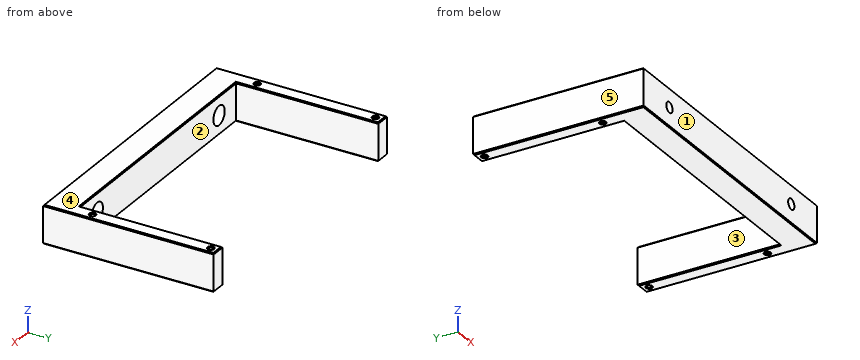
```python
from build123d import *

# Parameters (mm, degrees)
BOSS_EXTRUDE1_DEPTH            = 20
M3X0_5_TAPPED_HOLE1_D          = 2.5
CHAMFER1_SIZE                  = 0.5
CBORE_FOR_M5_SHCS1_D           = 5.5
CBORE_FOR_M5_SHCS1_CBORE_D     = 10
CBORE_FOR_M5_SHCS1_CBORE_DEPTH = 10


with BuildPart() as part:
    # Sketch2 → Boss-Extrude1 (new body)
    with BuildSketch(Plane.XY):
        Polygon((-76.2, 34.925), (-68.58, 34.925), (-68.58, -39.925), (68.58, -39.925), (68.58, 34.925), (76.2, 34.925), (76.2, -54.925), (-76.2, -54.925), align=None)
    extrude(amount=BOSS_EXTRUDE1_DEPTH)

    # M3x0.5 Tapped Hole1 (through all)
    with Locations(Plane(origin=(0, 0, 0), x_dir=(-1, 0, 0), z_dir=(0, 0, -1))):
        with Locations((-72.39, -31.115), (-72.39, 31.115), (72.39, 31.115), (72.39, -31.115)):
            Hole(M3X0_5_TAPPED_HOLE1_D / 2)

    # Chamfer1
    chamfer1_edges = [part.edges().sort_by_distance(p)[0] for p in [
        (72.39, 34.925, 0),
        (76.2, -10, 0),
        (0, -54.925, 0),
        (-76.2, -10, 0),
        (76.2, -10, 20),
        (72.39, 34.925, 20),
        (68.58, -2.5, 20),
        (0, -39.925, 20),
        (-73.64, -31.115, 0),
        (-73.64, -31.115, 20),
        (-68.58, -2.5, 20),
        (-73.64, 31.115, 0),
        (-73.64, 31.115, 20),
        (-72.39, 34.925, 20),
        (71.14, 31.115, 0),
        (71.14, 31.115, 20),
        (71.14, -31.115, 0),
        (71.14, -31.115, 20),
        (-76.2, -10, 20),
        (-72.39, 34.925, 0),
        (0, -54.925, 20),
        (-68.58, -2.5, 0),
        (0, -39.925, 0),
        (68.58, -2.5, 0),
    ]]
    chamfer(chamfer1_edges, length=CHAMFER1_SIZE)

    # CBORE for M5 SHCS1 (through all)
    with Locations(Plane(origin=(-53.58, -39.925, 10), x_dir=(1, 0, 0), z_dir=(0, 1, 0))):
        with Locations((0, 0), (107.16, 0)):
            CounterBoreHole(CBORE_FOR_M5_SHCS1_D / 2, CBORE_FOR_M5_SHCS1_CBORE_D / 2, CBORE_FOR_M5_SHCS1_CBORE_DEPTH)


solid = part.part
```
The model under review builds one solid part; all positions refer to its coordinate system, in mm. Face numbers are marked on the shaded views. A direction names the side the tool comes from. Round coordinates to 2 decimals unless told otherwise and drop trailing zeros. Order: outer loops, then holes, each group sorted by start corner. A loop starts at its lowest first (then second) coordinate and runs counter-clockwise, first axis right, second up. Notation, with made-up numbers: (65.5, -30) -> (83.5, -30) arc R26 cw to (83.5, -2) -> close; hole circle Ø3 at (-18.5, 68.5). An arc over 180 degrees is marked (long way). One line per item, written item: value. Start each with the question number.
Q1. Take a section at B-B (x = -53.58). Write out the cut boundary in (y, z) (3 decimals), and give its area (3 significant figures).
Q2. Wall thickness on line 1 (X direction, y = -53.5, z = 10); line 2 (Y direction, x = -72.39, z = 10.25) (3 decimals); line 3 (Z direction, x = 53.58, y = -45.75): over which ranges is each line inside the solid? List them lowest first.
Q3. Mouldability with a two-part tool opening along X and no side actions: class the marked faces 3, 4 and 5 as released by +X, released by -X, zero draft, split by the parting line, or undercut.
Q4. Take a section at D-D (x = 35). Write out the cut boundary in (y, z) (3 decimals), and give its area (4 significant figures).
Q5. Take a section at A-A (y = -35). Write out the cut boundary in (x, z), and give its area (3 significant figures).
Q6. Take a section at C-C (z = 10). Write out the cut boundary in (x, y) (3 decimals).
Q7. Machinability: for the marked faces 1 and 2, which of the approach directions +Z, -Z, +X, -X, +Y, -Y give a long, thin tool a straight path to every point of the face, cutting with its end or side? Answer none if there is none.
Q8. Clearance check with flat-ended pins moving along their axes: pin 1 Ø5 at (x, z) = (-53.5, 11) entering from +Y (3 decimals); pin 2 Ø1.5 at (x, y) = (72.39, -31.115) entering from -Z; pin 3 Ø11 at (x, z) = (51, 10.5) entering from +Y (3 decimals); pin 4 Ø9 at (x, z) = (53.58, 10) entering from -Y (3 decimals). State where each tip first meets the part, or that it passes through.
Reported:
1. outline: (-54.925, 0.5) -> (-54.425, 0) -> (-40.425, 0) -> (-39.925, 0.5) -> (-39.925, 5) -> (-49.925, 5) -> (-49.925, 7.25) -> (-54.925, 7.25) -> close; (-54.925, 12.75) -> (-49.925, 12.75) -> (-49.925, 15) -> (-39.925, 15) -> (-39.925, 19.5) -> (-40.425, 20) -> (-54.425, 20) -> (-54.925, 19.5) -> close
1. area: 172 mm2
2. line 1: x = -76.2 to -56.33, -50.83 to 50.83, 56.33 to 76.2
2. line 2: y = -54.925 to -32.365, -29.865 to 29.865, 32.365 to 34.925
2. line 3: z = 0 to 5, 15 to 20
3. face 3: undercut
3. face 4: zero draft
3. face 5: released by -X
4. outline: (-54.925, 0.5) -> (-54.425, 0) -> (-40.425, 0) -> (-39.925, 0.5) -> (-39.925, 19.5) -> (-40.425, 20) -> (-54.425, 20) -> (-54.925, 19.5) -> close
4. area: 299.5 mm2
5. outline: (-76.2, 0.5) -> (-75.7, 0) -> (-69.08, 0) -> (-68.58, 0.5) -> (-68.58, 19.5) -> (-69.08, 20) -> (-75.7, 20) -> (-76.2, 19.5) -> close; (68.58, 0.5) -> (69.08, 0) -> (75.7, 0) -> (76.2, 0.5) -> (76.2, 19.5) -> (75.7, 20) -> (69.08, 20) -> (68.58, 19.5) -> close
5. area: 304 mm2
6. outline: (-76.2, -54.925) -> (-56.33, -54.925) -> (-56.33, -49.925) -> (-58.58, -49.925) -> (-58.58, -39.925) -> (-68.58, -39.925) -> (-68.58, 34.925) -> (-76.2, 34.925) -> close; (-50.83, -54.925) -> (50.83, -54.925) -> (50.83, -49.925) -> (48.58, -49.925) -> (48.58, -39.925) -> (-48.58, -39.925) -> (-48.58, -49.925) -> (-50.83, -49.925) -> close; (56.33, -54.925) -> (76.2, -54.925) -> (76.2, 34.925) -> (68.58, 34.925) -> (68.58, -39.925) -> (58.58, -39.925) -> (58.58, -49.925) -> (56.33, -49.925) -> close; hole circle Ø2.5 at (-72.39, -31.115); hole circle Ø2.5 at (-72.39, 31.115); hole circle Ø2.5 at (72.39, -31.115); hole circle Ø2.5 at (72.39, 31.115)
7. face 1: +Z, -Z, +X, -X, -Y
7. face 2: +Z, -Z, +Y
8. pin 1: stops at y = -49.925
8. pin 2: passes through
8. pin 3: stops at y = -39.925
8. pin 4: stops at y = -54.925
